```python
from build123d import *

# Parameters (mm, degrees)
FILLET3_R = 1.7
FILLET4_R = 1.7


with BuildPart() as part:
    # Sketch1 → Revolve2 (revolve)
    with BuildSketch(Plane.XY, mode=Mode.PRIVATE) as revolve2_sk:
        Polygon((-3.114208506, -0.827200396), (7.306092253, -0.827200396), (7.306092253, -14.720657828), (3.953440281, -14.720657828), (3.953440281, -6.120657828), (-1.56177698, -6.120657828), (-1.56177698, -13.020657828), (-25.583612163, -13.020657828), (-25.583612163, -6.120657828), (-8.302598077, -6.120657828), (-8.302598077, 0.602670746), (-3.114208506, 0.602670746), align=None)
    revolve(revolve2_sk.sketch.rotate(Axis((38.306092253, 0.602670746, 0), (0, -1, 0)), 270), axis=Axis((38.306092253, 0.602670746, 0), (0, -1, 0)))

    # Fillet3
    # the kernel refuses this fillet: 1.7 mm, written as the material it adds along each edge
    with BuildSketch(Plane(origin=(38.306092253, -0.827200396, 0), x_dir=(0, 0, 1), z_dir=(1, 0, 0))) as fillet3_piece_1:
        with BuildLine():
            CenterArc((39.741899614, -1.7), FILLET3_R, 9.143015085, 80.856984915)
            Line((41.420300758, -1.429871142), (41.453868781, -1.424468565))
            ThreePointArc((41.453868781, -1.424468565), (41.454300758, -0.714935571), (41.454300758, 0))
            Line((41.454300758, 0), (41.420300758, 0.034))
            Line((41.420300758, 0.034), (39.741899614, 0.034))
            Line((39.741899614, 0.034), (39.741899614, 0))
        make_face()
    revolve(axis=Axis((38.306092253, -0.827200396, 0), (0, -1, 0)))

    # Fillet4
    fillet4_edges = [part.edges().sort_by_distance(p)[0] for p in [
        (38.306092253, -13.020657828, -63.889704416),
    ]]
    fillet(fillet4_edges, radius=FILLET4_R)


solid = part.part
```
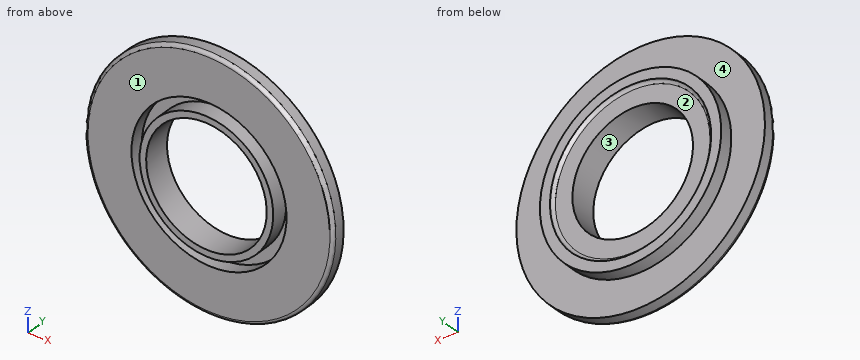
CAD build for the part. Positions are in the model's coordinates, mm. Face numbers are marked on the shaded views. A direction names the side the tool comes from. Round coordinates to 2 decimals unless told otherwise and drop trailing zeros. Write each loop counter-clockwise with the first axis right and the second up, starting at its lowest first coordinate (ties: lowest second). Pieces come first, ordered by that corner, then holes.
Item 1: Band-saw the part on A-A on z = 0. Write the cut outline in (x, y).
Filled in:
outline: (-25.58, -11.32) arc R1.7 ccw to (-23.88, -13.02) - (-1.56, -13.02) - (-1.56, -6.12) - (3.95, -6.12) - (3.95, -14.72) - (7.31, -14.72) - (7.31, -0.83) - (-1.44, -0.83) arc R1.7 cw to (-3.11, 0.6) - (-8.3, 0.6) - (-8.3, -6.12) - (-25.58, -6.12) - close; (69.31, -14.72) - (72.66, -14.72) - (72.66, -6.12) - (78.17, -6.12) - (78.17, -13.02) - (100.5, -13.02) arc R1.7 ccw to (102.2, -11.32) - (102.2, -6.12) - (84.91, -6.12) - (84.91, 0.6) - (79.73, 0.6) arc R1.7 cw to (78.05, -0.83) - (69.31, -0.83) - close
Item 2: Drop flat-ended pins along their axis: pin 1 Ø1 at (y, z) = (-11.5, 0.5) entering from -X; pin 2 Ø1 at (x, z) = (1, 45.5) entering from +Y; pin 3 Ø5 at (x, y) = (62.5, -5.5) entering from -Z. Give the stop position or say it passes through.
Filled in:
pin 1: stops at x = -25.58
pin 2: stops at y = -6.12
pin 3: stops at z = -60.07
Item 3: Drill centre lines: L1, parallel to X at y = -10.25, z = 0; L2, parallel to X at y = -4.5, z = 0; L3, parallel to X at y = -10, z = -3. Where is each one in solid material? Low to high.
Filled in:
L1: x = -25.58 to -1.56, 3.95 to 7.31, 69.31 to 72.66, 78.17 to 102.2
L2: x = -8.3 to 7.31, 69.31 to 84.91
L3: x = -25.51 to -1.45, 4.08 to 7.45, 69.16 to 72.53, 78.06 to 102.13
Item 4: Band-saw the part on B-B on y = -2.75. Write the cut outline in (x, z), then the cut area to 3 significant figures.
Filled in:
outline: circle Ø93.22 at (38.31, 0); hole circle Ø62 at (38.31, 0)
area: 3,810 mm2
Item 5: Mould opens along X. For the marked faces 3 and 4 say: released by +X, released by -X, zero draft, split by the parting line, or undercut.
Filled in:
face 3: undercut
face 4: zero draft
Item 6: Band-saw the part on C-C on y = -9.25. Write the cut outline in (x, z), then the cut area to 3 significant figures.
Filled in:
outline: circle Ø127.78 at (38.31, 0); circle Ø68.71 at (38.31, 0); hole circle Ø79.74 at (38.31, 0); hole circle Ø62 at (38.31, 0)
area: 8,520 mm2
Item 7: Tool access for the marked faces 1 and 2: list every direction of +Z, -Z, +X, -X, +Y, -Y with a clear straight run to the whole face (end or side of a thin tool).
Filled in:
face 1: -Y
face 2: +Y
